```python
from build123d import *

# Parameters (mm, degrees)
SKETCH3_W          = 1.27
SKETCH3_H          = 10.683807707
CUT_EXTRUDE1_DEPTH = 1.6002


with BuildPart() as part:
    # Sketch1 → Revolve1 (revolve)
    with BuildSketch(Plane.XY):
        Polygon((0, 0), (0, 3.7465), (6.0198, 3.7465), (6.0198, 5.08), (7.62, 5.08), (7.62, 0), align=None)
    revolve(axis=Axis((7.62, 0, 0), (-1, 0, 0)))

    # Sketch3 → Cut-Extrude1 (cut)
    with BuildSketch(Plane(origin=(7.62, 0, 0), x_dir=(0, 0, -1), z_dir=(1, 0, 0))):
        with Locations((0, -0.049309881)):
            Rectangle(SKETCH3_W, SKETCH3_H)
    extrude(amount=-CUT_EXTRUDE1_DEPTH, mode=Mode.SUBTRACT)


solid = part.part
```
Here's how the part is built. I have some questions about the finished solid (model axes, mm). A direction names the side the tool comes from. Coordinates: 2 decimals unless noted, no trailing zeros. Loops run counter-clockwise (first coordinate to the right, second up) from the corner with the lowest first, then second, coordinate; pieces in that order, holes last. Notation, with made-up numbers: (24.25, 44.5) -> (83.25, 44.5) arc R5 ccw to (83.25, 48.5) -> close; hole circle Ø10 at (52, 80). An arc over 180 degrees is marked (long way). Return JSON: item names as keys, results as strings.
1) If we section it at C-C, the plane y = -4: Write out the boundary of the cut face in (x, z) (3 decimals), then the cut area to 3 significant figures.
Results below:
{"outline": "(6.02, -3.132) -> (7.62, -3.132) -> (7.62, -0.635) -> (6.02, -0.635) -> close; (6.02, 0.635) -> (7.62, 0.635) -> (7.62, 3.132) -> (6.02, 3.132) -> close", "area": "7.99 mm²"}
2) If we section it at B-B, the plane z = 1: Write out the boundary of the cut face in (x, y), then the cut area to 3 significant figures.
Results below:
{"outline": "(0, -3.61) -> (6.02, -3.61) -> (6.02, -4.98) -> (7.62, -4.98) -> (7.62, 4.98) -> (6.02, 4.98) -> (6.02, 3.61) -> (0, 3.61) -> close", "area": "59.4 mm²"}
3) If we section it at D-D, the plane x = 6.5: Write out the boundary of the cut face in (y, z) (3 decimals).
Results below:
{"outline": "(-5.04, -0.635) arc R5.08 ccw to (5.04, -0.635) -> close; (-5.04, 0.635) -> (5.04, 0.635) arc R5.08 ccw to start"}
4) I need wall thicknesses on line 1 (X direction, y = -2, z = 0.25); line 2 (Z direction, x = 2, y = 0); line 3 (Z direction, x = 7, y = -2) (3 decimals). Which ranges of each line are inside material? Lowest first, please. Write a range as from..to.
Results below:
{"line 1": "0..6.02", "line 2": "-3.75..3.75", "line 3": "-4.67..-0.635, 0.635..4.67"}
5) If we section it at A-A, the plane y = 0: Write out the boundary of the cut face in (x, z) (1 decimal).
Results below:
{"outline": "(0, -3.7) -> (6, -3.7) -> (6, -5.1) -> (7.6, -5.1) -> (7.6, -0.6) -> (6, -0.6) -> (6, 0.6) -> (7.6, 0.6) -> (7.6, 5.1) -> (6, 5.1) -> (6, 3.7) -> (0, 3.7) -> close"}
6) Will these pins go through, and if not, where does the flat tip stop? pin 1 (1.3 mm diameter, centred on x = 6.5, y = 1.5, fed in from -Z); pin 2 (1.3 mm diameter, centred on x = 6.5, y = -2, fed in from +Z); pin 3 (2 mm diameter, centred on x = 4, y = -1.5, fed in from +Z).
Results below:
{"pin 1": "z = -5.01", "pin 2": "z = 4.9", "pin 3": "z = 3.71"}
7) Thinking about a two-plate mould opening in Z: for faces 1 (the face through (7.62, 0, -2)), 2 (the face through (6.02, 0, 0)), 3 (the face through (6.83, -0.1, 5.08)), which applies, +Z half, -Z half, draft (parallel to the pull), parting line (faces both ways), or undercut?
Results below:
{"face 1": "draft", "face 2": "undercut", "face 3": "+Z half"}
8) For faces 4 (the face through (6.02, 0, -4)), 5 (the face through (7, 0, 0.635)), 6 (the face through (3.052, -0.488, -3.715)), 7 (the face through (6.02, 0, 4)), 8 (the face through (6.83, 0.1, -5.08)), which set-ups out of +Z, -Z, +X, -X, +Y, -Y let a thin tool reach every point of the face, with its end or its side?
Results below:
{"face 4": "-Z, -X", "face 5": "+X, +Y, -Y", "face 6": "-X", "face 7": "+Z, -X", "face 8": "-Z, +X, -X"}
